Autodesk Inventor part; units mm, degrees
ref_plane "YZ Plane" through (0, 0, 0) normal (1, 0, 0) x (0, 1, 0)
ref_plane "XZ Plane" through (0, 0, 0) normal (0, 1, 0) x (-1, 0, 0)
ref_plane "XY Plane" through (0, 0, 0) normal (0, 0, 1) x (1, 0, 0)
sketch "Sketch1" plane through (0, 0, 0) normal (0, 0, 1) x (1, 0, 0)
  line L0 (0, 0) -> (31.75, 0)
  line L1 (31.75, 0) -> (31.75, 20.32)
  line L2 (31.75, 20.32) -> (0, 20.32)
  line L3 (0, 20.32) -> (0, 0)
  circle A0 centre (15.875, 10.16) radius 9.2075
  dimension "d0" = 20.32
  dimension "d1" = 31.75
  dimension "d2" = 15.875
  dimension "d3" = 15.875
  dimension "d4" = 10.16
  dimension "d5" = 10.16
  dimension "d6" = 18.415
extrude "Extrusion1" add sketch "Sketch1" along normal blind 2.032
chamfer "Chamfer2" distance 2.032 angle 45 2 edges at (0, 10.16, 2.032) (31.75, 10.16, 2.032)
sketch "Sketch2" plane through (0, 0, 2.032) normal (0, 0, 1) x (1, 0, 0)
  line L0 (14.224, 21.0828) -> (17.526, 21.0828)
  line L1 (17.526, 21.0828) -> (17.526, 18.4625)
  line L2 (17.526, 18.4625) -> (14.224, 18.4625)
  line L3 (14.224, 18.4625) -> (14.224, 21.0828)
  line L4 (2.032, 0) -> (2.032, 20.32)
  line L5 (29.718, 20.32) -> (29.718, 0)
  point P0 (0, 0)
  point P1 (14.224, 19.7726)
  dimension "d15" = 12.192
  dimension "d16" = 12.192
extrude "Extrusion2" cut sketch "Sketch2" against normal blind 0.762
properties part number "org_case_psu_connector"
Geometry: final body of the model. Coordinates: model frame, mm. Give positions to 0.01 mm unless a question says otherwise; leave off trailing zeros. Loops run counter-clockwise (first coordinate to the right, second up) from the corner with the lowest first, then second, coordinate; pieces in that order, holes last. Notation, with made-up numbers: M 39.25,50.25 L 67.25,50.25 A22 ccw 67.25,70.25 Z; hole C 33.5,-1.5 d11. An arc over 180 degrees is marked long. Put each result on its own line as item: value. Start each with the question number.
1) Contact query for flat-ended pins moving along their axis: pin 1 (4 mm diameter, centred on x = 23.5, y = 12, fed in from +Z); pin 2 (11 mm diameter, centred on x = 15.875, y = 10.16, fed in from +Z); pin 3 (0.8 mm diameter, centred on y = 19.5, z = 1.5, fed in from -X); pin 4 (0.8 mm diameter, centred on y = 19.5, z = 2, fed in from +X). Output: stop coordinate, or through.
2) Ray query, line 1 along X through (y, z) = (11.75, 0.25); line 2 along Y through (x, z) = (8, 1.15); line 3 along X through (y, z) = (13.5, 1.2). Return the intervals inside material, ascending.
3) Cut plane D-D (x = 24.5). Output: boundary loops of the cut face in (y, z).
4) Cut plane B-B (x = 16.5). Output: boundary loops of the cut face in (y, z).
5) Pull-direction query (Y, two-part tool) for faces 1 (the flat face through (16, 0, 1)), 2 (the cylindrical face through (24.38, 13.69, 1)), 3 (the flat face through (16, 20.32, 1)), 4 (the flat face through (16, 20, 1.27)); classes: pulls with the +Y half, pulls with the -Y half, needs draft (parallel to the pull), parting line crosses it, or undercut.
Verdict:
1. pin 1: z = 2.03
1. pin 2: through
1. pin 3: x = 1.1
1. pin 4: x = 30.15
2. line 1: 0.25 to 6.81, 24.94 to 31.5
2. line 2: 0 to 5.39, 14.93 to 20.32
2. line 3: 1.2 to 7.29, 24.46 to 30.55
3. outline: M 0,0 L 6.94,0 L 6.94,2.03 L 0,2.03 Z; M 13.38,0 L 20.32,0 L 20.32,2.03 L 13.38,2.03 Z
4. outline: M 0,0 L 0.97,0 L 0.97,2.03 L 0,2.03 Z; M 19.35,0 L 20.32,0 L 20.32,1.27 L 19.35,1.27 Z
5. face 1: pulls with the -Y half
5. face 2: undercut
5. face 3: pulls with the +Y half
5. face 4: needs draft
